Answer from the drawing. Dimensions are ordinates in mm from the lowest x, y and z of the part. Give positions to 0.01 mm unless a question says otherwise; leave off trailing zeros. Order: outer loops, then holes, each group sorted by start corner. A loop starts at its lowest first (then second) coordinate and runs counter-clockwise, first axis right, second up. Notation, with made-up numbers: (31, -16) - (57, -16) arc R20 cw to (57, -12) - close; hole circle Ø6 at (-4, -7.75). An arc over 180 degrees is marked (long way). Write each question's results on one line, items separated by ' | '.
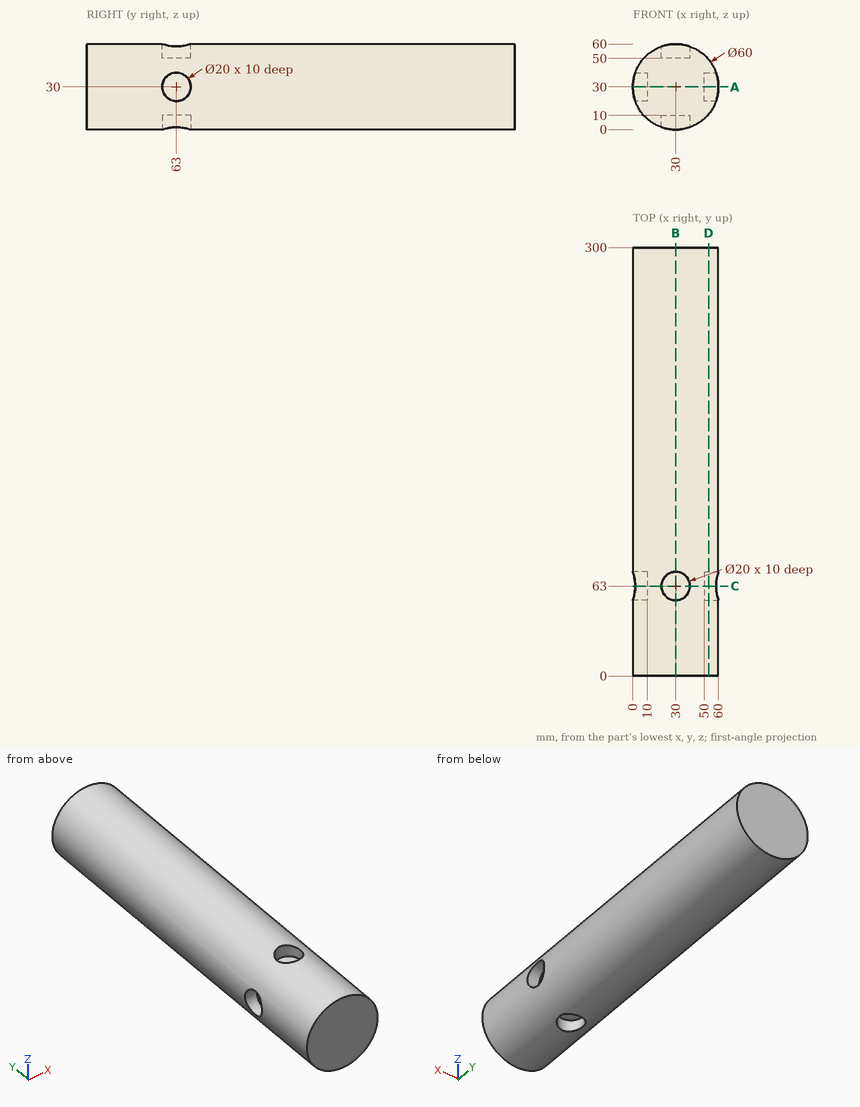
1. A cutting plane is placed at D-D, the plane x = 53. Write down the section's boundary in (y, z).
Answer list:
outline: (0, 10.74) - (300, 10.74) - (300, 49.26) - (0, 49.26) - close; hole circle Ø20 at (63, 30)
2. A cutting plane is placed at B-B, the plane x = 30. Write down the section's boundary in (y, z).
Answer list:
outline: (0, 0) - (53, 0) - (53, 10) - (73, 10) - (73, 0) - (300, 0) - (300, 60) - (73, 60) - (73, 50) - (53, 50) - (53, 60) - (0, 60) - close
3. A cutting plane is placed at C-C, the plane y = 63. Write down the section's boundary in (x, z), then the cut area to 3 significant figures.
Answer list:
outline: (1.72, 20) arc R30 ccw to (20, 1.72) - (20, 10) - (40, 10) - (40, 1.72) arc R30 ccw to (58.28, 20) - (50, 20) - (50, 40) - (58.28, 40) arc R30 ccw to (40, 58.28) - (40, 50) - (20, 50) - (20, 58.28) arc R30 ccw to (1.72, 40) - (10, 40) - (10, 20) - close | area: 2,070 mm^2
4. Given P1, Ø6, axis at y = 60.5, z = 33, coming from the -X side; P2, Ø5, axis at x = 17, y = 258, coming from the -Z side; P3, Ø10, axis at y = 67, z = 26, coming from the +X side, each flat-ended and moving along its own axis, determine where each tip first touches the part or whether it passes through.
Answer list:
P1: x = 10 | P2: z = 1.9 | P3: x = 59.68
5. A cutting plane is placed at A-A, the plane z = 30. Write down the section's boundary in (x, y).
Answer list:
outline: (0, 0) - (60, 0) - (60, 53) - (50, 53) - (50, 73) - (60, 73) - (60, 300) - (0, 300) - (0, 73) - (10, 73) - (10, 53) - (0, 53) - close
6. Straight lines are drawn through the part: line 1 (Y direction, x = 56, z = 30); line 2 (Y direction, x = 51, z = 29); line 3 (X direction, y = 180, z = 31). For each, find the intervals that lie inside material, in ascending order. Write a range as [from, to].
Answer list:
line 1: [0, 53], [73, 300] | line 2: [0, 53.05], [72.95, 300] | line 3: [0.02, 59.98]
